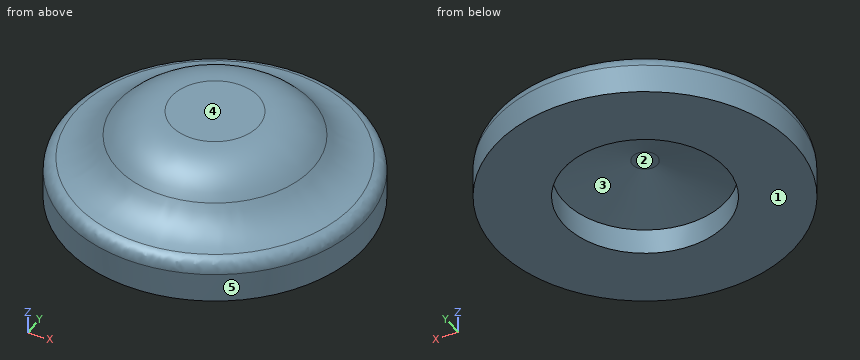
```python
from build123d import *

# Parameters (mm, degrees)
F4_R     = 1
F5_R     = 5.9
F6_DEPTH = 2.85
F7_SIZE2 = 1
F7_SIZE  = 5


# Not quite as in the source:
# - a fillet or chamfer that OpenCascade refuses, or shapes differently, is made with other operations: its cross-section is extruded or revolved along the edge and cut away or added


with BuildPart() as f1:
    # F0 (on Front) → F1 (revolve)
    with BuildSketch(Plane.XZ):
        Polygon((8, 13.6877541882), (0, 13.6877541882), (0, 6.9177541882), (10.85, 6.9177541882), (10.85, 9.9177541882), (8, 9.9177541882), align=None)
    revolve(axis=Axis((0, 0, 10.3027541882), (0, 0, 1)))

    # F2: fillet of radius 5 on 1 edges, made by hand

    # F2_s1 → F2_t2 (revolve, cut)
    with BuildSketch(Plane.XZ):
        with BuildLine():
            ThreePointArc((3.1536508586, 13.6877541882), (6.2236671452, 12.6342716403), (8, 9.9177541882))
            Line((8, 9.9177541882), (8, 13.6877541882))
            Line((8, 13.6877541882), (3.1536508586, 13.6877541882))
        make_face()
    revolve(axis=Axis((0, 0, 13.6877541882), (0, 0, 1)), mode=Mode.SUBTRACT)

    # F3: fillet of radius 5 on 1 edges, made by hand

    # F3_s1 → F3_t2 (revolve)
    with BuildSketch(Plane.XZ):
        with BuildLine():
            ThreePointArc((7.0654038886, 11.8019456133), (8.7487622666, 10.4401726424), (10.85, 9.9177541882))
            Line((10.85, 9.9177541882), (8, 9.9177541882))
            ThreePointArc((8, 9.9177541882), (7.6328955207, 10.9095478909), (7.0654038886, 11.8019456133))
        make_face()
    revolve(axis=Axis((0, 0, 9.9177541882), (0, 0, 1)))

    # F4
    f4_edges = [f1.edges().sort_by_distance(p)[0] for p in [
        (-10.85, 0, 9.917754),
    ]]
    fillet(f4_edges, radius=F4_R)

    # F5 (on face) → F6 (cut)
    with BuildSketch(Plane(origin=(0, 0, 6.9177541882), x_dir=(1, 0, 0), z_dir=(0, 0, -1))):
        Circle(F5_R)
    extrude(amount=-F6_DEPTH, mode=Mode.SUBTRACT)

    # F7
    f7_edges = [f1.edges().sort_by_distance(p)[0] for p in [
        (-5.9, 0, 9.767754),
    ]]
    f7_side = f1.faces().sort_by_distance((0, 0, 9.767754))[0]
    chamfer(f7_edges, length=F7_SIZE, length2=F7_SIZE2, reference=f7_side)


solid = f1.part
```
Check sheet for the modelled part. Datum: model origin and axes. Units: mm. Face numbers are marked on the shaded views. A direction names the side the tool comes from. Round coordinates to 2 decimals unless told otherwise and drop trailing zeros. Order: outer loops, then holes, each group sorted by start corner. A loop starts at its lowest first (then second) coordinate and runs counter-clockwise, first axis right, second up. Notation, with made-up numbers: (25.5, 43) - (83.5, 43) arc R28 ccw to (83.5, 74) - close; hole circle Ø9 at (-36, -31). An arc over 180 degrees is marked (long way). Answer as CSV lines item,"result". Start each with the question number.
1) Depth check by flat-ended pin: pin 1 (0.9 mm diameter, centred on x = -0.5, y = 0, fed in from -Z). Enter the tip coordinate at first touch or a pass-through.
2) Draft check along Y on the marked faces 3, 4 and 5. Enter one of: +Y half, -Y half, draft (parallel to the pull), parting line (faces both ways), or undercut.
3) Tool access check on the marked faces 1 and 2. Record the directions out of +Z, -Z, +X, -X, +Y, -Y that give a thin tool (end or side, any length) a straight path to the whole face; none if there is none.
4) Section check A-A (z = 8.25). Record the cut outline in (x, y), then the cut area to 3 significant figures.
5) Section check B-B (z = 10.5). Record the cut outline in (x, y), then the cut area to 3 significant figures.
6) Scan lines: probe 1 along X at (y, z) = (0, 8.3); probe 2 along Z at (x, y) = (-0.25, 0). Record each from-to range of solid material in increasing order.
Determined:
1,pin 1,"z = 9.76"
2,face 3,"undercut"
2,face 4,"draft"
2,face 5,"parting line"
3,face 1,"-Z, +X, -X, +Y, -Y"
3,face 2,"-Z"
4,outline,"circle Ø21.7 at (0, 0); hole circle Ø11.8 at (0, 0)"
4,area,"260 mm^2"
5,outline,"circle Ø17.26 at (0, 0)"
5,area,"234 mm^2"
6,probe 1,"-10.85 to -5.9, 5.9 to 10.85"
6,probe 2,"9.77 to 13.69"
